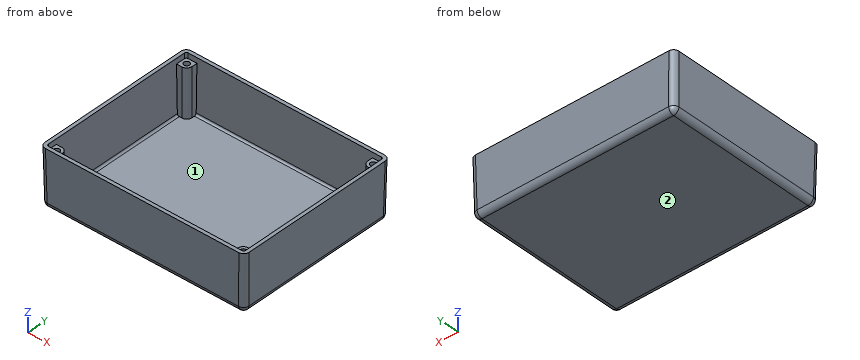
```python
from build123d import *

# Parameters (mm, degrees)
SKETCH1_W                       = 119.634
SKETCH1_H                       = 95.25
BOSS_EXTRUDE1_DEPTH             = 33.02
BOSS_EXTRUDE1_DRAFT             = -1
FILLET1_R                       = 3.175
SHELL1_T                        = -2.032
BOSS_EXTRUDE2_DEPTH             = 27.94
TAP_DRILL_FOR_M4X0_7_TAP1_D     = 3.3
TAP_DRILL_FOR_M4X0_7_TAP1_DEPTH = 25.4
TAP_DRILL_FOR_M4X0_7_TAP1_TIP   = 0.991420021


with BuildPart() as part:
    # Sketch1 → Boss-Extrude1 (with draft: the straight prism first)
    with BuildSketch(Plane.XY):
        with Locations((59.817, 47.625)):
            Rectangle(SKETCH1_W, SKETCH1_H)
    extrude(amount=-BOSS_EXTRUDE1_DEPTH)
    # Boss-Extrude1: the draft: its side faces are tilted about the plane it starts from
    boss_extrude1_sides = [part.faces().sort_by_distance(p)[0] for p in [
        (59.817, 0, -16.51),
        (119.634, 47.625, -16.51),
        (59.817, 95.25, -16.51),
        (0, 47.625, -16.51),
    ]]
    draft(boss_extrude1_sides, Plane.XY, BOSS_EXTRUDE1_DRAFT)

    # Fillet1
    fillet1_edges = [part.edges().sort_by_distance(p)[0] for p in [
        (119.057633756, 47.625, -33.02),
        (59.817, 94.673633756, -33.02),
        (0.576366244, 47.625, -33.02),
        (59.817, 0.576366244, -33.02),
        (0.288183122, 94.961816878, -16.51),
        (119.345816878, 94.961816878, -16.51),
        (119.345816878, 0.288183122, -16.51),
        (0.288183122, 0.288183122, -16.51),
    ]]
    fillet(fillet1_edges, radius=FILLET1_R)

    # Shell1
    shell1_openings = [part.faces().sort_by_distance(p)[0] for p in [
        (59.817, 47.625, 0),
    ]]
    offset(amount=SHELL1_T, openings=shell1_openings, kind=Kind.INTERSECTION)

    # Sketch2 → Boss-Extrude2 (add)
    with BuildSketch(Plane.XY.offset(-30.988)):
        with BuildLine():
            Line((2.032309531, 86.867690469), (5.207309531, 86.867690469))
            ThreePointArc((5.207309531, 86.867690469), (7.452373561, 87.797626439), (8.382309531, 90.042690469))
            Line((8.382309531, 90.042690469), (8.382309531, 93.217690469))
            Line((8.382309531, 93.217690469), (3.175135446, 93.217690469))
            ThreePointArc((3.175135446, 93.217690469), (2.367035492, 92.882964508), (2.032309531, 92.074864554))
            Line((2.032309531, 92.074864554), (2.032309531, 86.867690469))
        make_face()
        with BuildLine():
            Line((111.251690469, 93.217690469), (111.251690469, 90.042690469))
            ThreePointArc((111.251690469, 90.042690469), (112.181626439, 87.797626439), (114.426690469, 86.867690469))
            Line((114.426690469, 86.867690469), (117.601690469, 86.867690469))
            Line((117.601690469, 86.867690469), (117.601690469, 92.074864554))
            ThreePointArc((117.601690469, 92.074864554), (117.266964508, 92.882964508), (116.458864554, 93.217690469))
            Line((116.458864554, 93.217690469), (111.251690469, 93.217690469))
        make_face()
        with BuildLine():
            Line((116.458864554, 2.032309531), (111.251690469, 2.032309531))
            Line((111.251690469, 2.032309531), (111.251690469, 5.207309531))
            ThreePointArc((111.251690469, 5.207309531), (112.181626439, 7.452373561), (114.426690469, 8.382309531))
            Line((114.426690469, 8.382309531), (117.601690469, 8.382309531))
            Line((117.601690469, 8.382309531), (117.601690469, 3.175135446))
            ThreePointArc((117.601690469, 3.175135446), (117.266964508, 2.367035492), (116.458864554, 2.032309531))
        make_face()
        with BuildLine():
            Line((2.032309531, 3.175135446), (2.032309531, 8.382309531))
            Line((2.032309531, 8.382309531), (5.207309531, 8.382309531))
            ThreePointArc((5.207309531, 8.382309531), (7.452373561, 7.452373561), (8.382309531, 5.207309531))
            Line((8.382309531, 5.207309531), (8.382309531, 2.032309531))
            Line((8.382309531, 2.032309531), (3.175135446, 2.032309531))
            ThreePointArc((3.175135446, 2.032309531), (2.367035492, 2.367035492), (2.032309531, 3.175135446))
        make_face()
    extrude(amount=BOSS_EXTRUDE2_DEPTH)

    # Tap Drill for M4x0.7 Tap1
    with Locations(Plane.XY.offset(-3.048)):
        with Locations((5.207309531, 90.042690469), (114.426690469, 90.042690469), (114.426690469, 5.207309531), (5.207309531, 5.207309531)):
            Hole(TAP_DRILL_FOR_M4X0_7_TAP1_D / 2, depth=TAP_DRILL_FOR_M4X0_7_TAP1_DEPTH)
            with Locations((0, 0, -(TAP_DRILL_FOR_M4X0_7_TAP1_DEPTH + TAP_DRILL_FOR_M4X0_7_TAP1_TIP / 2))):  # 118° drill point
                Cone(0, TAP_DRILL_FOR_M4X0_7_TAP1_D / 2, TAP_DRILL_FOR_M4X0_7_TAP1_TIP, mode=Mode.SUBTRACT)


solid = part.part
```
Verification items for the finished model (mm, model axes). Face numbers are marked on the shaded views. Round coordinates to 2 decimals unless told otherwise and drop trailing zeros. Write each loop counter-clockwise with the first axis right and the second up, starting at its lowest first coordinate (ties: lowest second). Pieces come first, ordered by that corner, then holes. Notation, with made-up numbers: (53.5, 77) -> (75.5, 77) arc R12 ccw to (75.5, 83) -> close; hole circle Ø6 at (34.5, -20). An arc over 180 degrees is marked (long way). Write each question's results on one line, items separated by ' | '. Start each with the question number.
1. Material ranges on probe 1 along Y at (x, z) = (23, -30); probe 2 along Y at (x, z) = (29, -29.5); probe 3 along Y at (x, z) = (6.5, -24), recorded low to high. Write a range as from..to.
2. Cross-section at B-B (x = 75). Enter the section's corners in (y, z) (3 decimals), then the cut area to 3 significant figures.
3. Draft check along Y on the marked faces 1 and 2. Enter one of: +Y half, -Y half, draft (parallel to the pull), parting line (faces both ways), or undercut.
4. Cross-section at C-C (z = -8). Count the separate pieces of the cut face and the enclosed holes in it, then the cut area to 3 significant figures.
5. Depth check by flat-ended pin: P1, Ø2, axis at x = 93, y = 17, coming from the +Z side; P2, Ø1.9, axis at x = 115, y = 4.5, coming from the +Z side; P3, Ø8, axis at y = 15, z = -15.5, coming from the +X side. Enter the tip coordinate at first touch or a pass-through.
6. Cross-section at A-A (y = 61). Enter the section's corners in (x, z) (3 decimals).
Solutions:
1) probe 1: y = 0.53..2.56, 92.69..94.72 | probe 2: y = 0.51..2.55, 92.7..94.74 | probe 3: y = 0.42..4.18, 6.23..8.11, 87.14..89.02, 91.07..94.83
2) outline: (0, 0) -> (0.522, -29.9) arc R3.175 ccw to (3.696, -33.02) -> (91.554, -33.02) arc R3.175 ccw to (94.728, -29.9) -> (95.25, 0) -> (93.218, 0) -> (92.696, -29.865) arc R1.143 cw to (91.554, -30.988) -> (3.696, -30.988) arc R1.143 cw to (2.554, -29.865) -> (2.032, 0) -> close | area: 314 mm2
3) face 1: undercut | face 2: draft
4) separate pieces: 1 | enclosed holes: 5 | area: 957 mm2
5) P1: stops at z = -30.99 | P2: stops at z = -3.05 | P3: stops at x = 119.43
6) outline: (0, 0) -> (0.522, -29.9) arc R3.175 ccw to (3.696, -33.02) -> (115.938, -33.02) arc R3.175 ccw to (119.112, -29.9) -> (119.634, 0) -> (117.602, 0) -> (117.08, -29.865) arc R1.143 cw to (115.938, -30.988) -> (3.696, -30.988) arc R1.143 cw to (2.554, -29.865) -> (2.032, 0) -> close
